Could you check a few things on this model? Use its own coordinates, in mm. Face numbers are marked on the shaded views. A direction names the side the tool comes from. Give positions to 0.01 mm unless a question says otherwise; leave off trailing zeros. Order: outer loops, then holes, each group sorted by start corner. A loop starts at its lowest first (then second) coordinate and runs counter-clockwise, first axis right, second up.
(1) If I drill on probe 1 along Y at (x, z) = (0, 5); probe 2 along Y at (x, z) = (-11.8, 11) (3 decimals); probe 3 along Z at (x, y) = (-6, -4), over which ranges is the centre line in solid material (lowest first)?
(2) On a 3-axis mill with a long thin cutter (end or side, diameter ignored), from which of +Z, -Z, +X, -X, +Y, -Y can I reach the whole of each face in a straight line? I mean the marked faces 5 and 6. Say none if no direction works.
(3) Imagine slicing it at A-A, the plane x = -4.5. Write out the boundary of the cut face in (y, z), then the cut area to 3 significant figures.
(4) If we mould it in two halves opening along Z, with no side actions, what happens to the marked faces 1, 2, 3 and 4? For each: released by +Z, released by -Z, zero draft, split by the parting line, or undercut.
(5) Will these pins go through, and if not, where does the flat tip stop? pin 1 (1 mm diameter, centred on x = -10, z = 13.5, fed in from +Y); pin 2 (1.8 mm diameter, centred on x = -5, z = 1.5, fed in from -Y); pin 3 (6.5 mm diameter, centred on x = -1, y = -1, fed in from +Z); pin 4 (2 mm diameter, centred on x = -9.5, z = 12, fed in from -Y) (3 decimals).
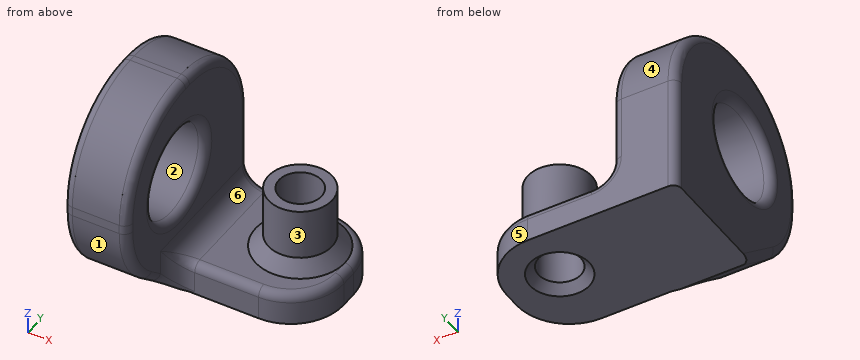
Autodesk Inventor part; units mm, degrees
ref_plane "YZ Plane" through (0, 0, 0) normal (1, 0, 0) x (0, 1, 0)
ref_plane "XZ Plane" through (0, 0, 0) normal (0, 1, 0) x (-1, 0, 0)
ref_plane "XY Plane" through (0, 0, 0) normal (0, 0, 1) x (1, 0, 0)
sketch "Эскиз1" plane through (0, 0, 0) normal (0, 0, 1) x (1, 0, 0)
  circle A0 centre (0, 0) radius 2
  circle A1 centre (0, 0) radius 5.625 construction
  line L0 (-14, -9.625) -> (5, -9.625) construction
  line L1 (5, -9.625) -> (5, -1.625) construction
  line L2 (-14, -1.625) -> (-14, -9.625) construction
  line L3 (-14, -5.625) -> (5, -5.625) construction
  line L4 (-14, -13.625) -> (5, -13.625)
  line L5 (5, -13.625) -> (5, 5)
  line L6 (-14, 5) -> (-14, -13.625)
  circle A2 centre (0, 0) radius 6.5 construction
  line L7 (-14, 5) -> (5, 5)
  line L8 (0, -17.65) -> (0, 10.525) construction
  line L9 (-8, 5) -> (-8, -13.625) construction
  line L10 (-18.1, 0) -> (10.6, 0) construction
  line L11 (-8, -13.625) -> (-8, -6.5)
  line L12 (-8, -6.5) -> (5, -6.5)
  dimension "d0" = 4
  dimension "d1" = 11.25
  dimension "d5" = 13
  dimension "d11" = 6
  dimension "d36" = 5
  dimension "d37" = 5
  dimension "d39" = 8
  dimension "d40" = 4
  dimension "d41" = 4
extrude "Выдавливание1" add sketch "Эскиз1" along normal blind 3 contours L6 L7 L5 L12 L11 L4
sketch "Эскиз3" plane through (0, 0, 3) normal (0, 0, 1) x (1, 0, 0)
  line L0 (-14, -13.625) -> (-8, -13.625)
  line L1 (-14, 5) -> (-8, 5)
  line L2 (-8, 5) -> (-8, -13.625)
  line L3 (-8, -13.625) -> (-14, -13.625)
  line L4 (-14, -13.625) -> (-14, 5)
  point P0 (0, 0)
  point P1 (5, -13.625)
  point P2 (4, 5)
  dimension "d17" = 6
extrude "Выдавливание3" add sketch "Эскиз3" along normal blind 17
sketch "Эскиз4" plane through (-14, -13.625, 0) normal (1, 0, 0) x (0, 0, -1)
  circle A0 centre (-11, 8) radius 4.3
  line L0 (0, 7.125) -> (0, 18.625)
  line L1 (0, 0) -> (-20, 0)
  line L2 (-20, 18.625) -> (-20, 0)
  line L3 (0, 18.625) -> (0, 0)
  line L4 (0, 7) -> (-6, 0)
  point P0 (0, 13.625)
  dimension "d20" = 8.6
  dimension "d42" = 9
  dimension "d48" = 8
  dimension "d49" = 7
  dimension "d50" = 6
extrude "Выдавливание4" cut sketch "Эскиз4" along normal up to surface (6 mm away)
sketch "Эскиз2" plane through (0, 0, 3) normal (0, 0, 1) x (1, 0, 0)
  circle A0 centre (0, 0) radius 3
  circle A1 centre (0, 0) radius 2
  dimension "d14" = 6
extrude "Выдавливание2" add sketch "Эскиз2" along normal blind 6
fillet "Сопряжение1" radius 9 3 edges at (-11, 5, 20) (-11, -13.625, 20) (-11, -13.625, 6)
fillet "Сопряжение1" radius 5 2 edges at (5, 5, 1.5) (5, -6.5, 1.5)
fillet "Сопряжение1" radius 2 2 edges at (-8, -6.5, 1.5) (-8, -0.75, 3)
chamfer "Фаска1" distance 1.2 angle 45 1 edges at (-3, 0, 3)
fillet "Сопряжение2" radius 0.8 9 edges at (-8, -5.625, 15.3) (-14, -5.625, 15.3) (-14, -13.625, 10.5697) (-14, 2.364, 17.364) (-8, 5, 8) (-8, -13.625, 10.5697) (-8, 2.364, 17.364) (-8, -9.4911, 2.4566) (-14, -8.5536, 1.6531)
chamfer "Фаска2" distance 0.8 angle 45 1 edges at (-2, 0, 0)
properties part number "Петля ролика"
Answer block:
1. probe 1: y = -3 to -2, 2 to 3
1. probe 2: y = -13.625 to -9.925, -1.325 to 5
1. probe 3: z = 0 to 3
2. face 5: +Z, -Z, +X, +Y
2. face 6: +Z, +Y, -Y
3. outline: (-6.5, 0) - (5, 0) - (5, 2.2) arc R0.8 ccw to (4.2, 3) - (-5.7, 3) arc R0.8 ccw to (-6.5, 2.2) - close
3. area: 34.2 mm2
4. face 1: released by -Z
4. face 2: undercut
4. face 3: zero draft
4. face 4: released by +Z
5. pin 1: stops at y = 4.77
5. pin 2: stops at y = -6.5
5. pin 3: stops at z = 9
5. pin 4: stops at y = -13.625
